The model under review builds one solid part; all positions refer to its coordinate system, in mm. Face numbers are marked on the shaded views. A direction names the side the tool comes from. Give positions to 0.01 mm unless a question says otherwise; leave off trailing zeros. Write each loop counter-clockwise with the first axis right and the second up, starting at its lowest first coordinate (ties: lowest second). Pieces come first, ordered by that corner, then holes. Notation, with made-up numbers: M 72,37 L 123,37 A7 ccw 123,46 Z; hole C 26.5,-21.75 d8. An arc over 180 degrees is marked long. Write item = value, one per line. Start each with the question number.
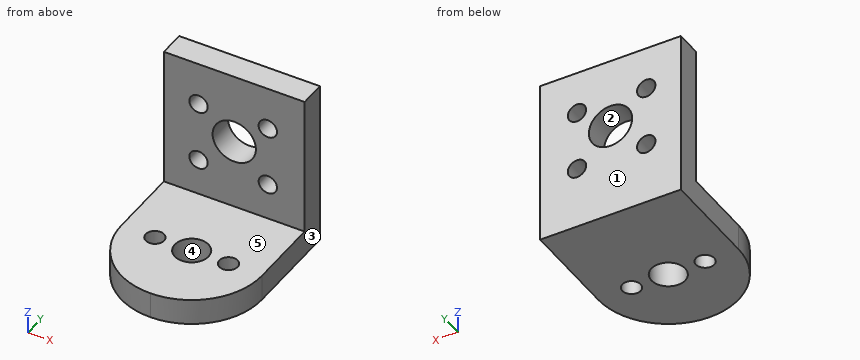
```python
from build123d import *

# Parameters (mm, degrees)
SKETCH1_W           = 32.5
SKETCH1_H           = 32.5
SKETCH1_R           = 2.125
SKETCH1_R_2         = 5
BOSS_EXTRUDE1_DEPTH = 6
SKETCH2_W           = 32.5
SKETCH2_H           = 6
BOSS_EXTRUDE2_DEPTH = 39
CUT_EXTRUDE1_DEPTH  = 39
SKETCH4_R           = 3.9
SKETCH4_R_2         = 2.125
CUT_EXTRUDE2_DEPTH  = 39


with BuildPart() as part:
    # Sketch1 → Boss-Extrude1 (new body)
    with BuildSketch(Plane(origin=(0, 0, 0), x_dir=(1, 0, 0), z_dir=(0, 1, 0))):
        with Locations((16.25, 16.25)):
            Rectangle(SKETCH1_W, SKETCH1_H)
        with Locations(Location((24, 10, 0), (0, 0, 270))):
            Circle(SKETCH1_R, mode=Mode.SUBTRACT)
        with Locations(Location((24, 24, 0), (0, 0, 270))):
            Circle(SKETCH1_R, mode=Mode.SUBTRACT)
        with Locations(Location((8, 24, 0), (0, 0, 270))):
            Circle(SKETCH1_R, mode=Mode.SUBTRACT)
        with Locations(Location((8, 10, 0), (0, 0, 270))):
            Circle(SKETCH1_R, mode=Mode.SUBTRACT)
        with Locations(Location((16.25, 16.25, 0), (0, 0, 270))):
            Circle(SKETCH1_R_2, mode=Mode.SUBTRACT)
    extrude(amount=BOSS_EXTRUDE1_DEPTH)

    # Sketch2 → Boss-Extrude2 (add)
    with BuildSketch(Plane(origin=(0, 6, 0), x_dir=(1, 0, 0), z_dir=(0, 1, 0))):
        with Locations((16.25, 35.5)):
            Rectangle(SKETCH2_W, SKETCH2_H)
    extrude(amount=-BOSS_EXTRUDE2_DEPTH)

    # Sketch3 → Cut-Extrude1 (cut)
    with BuildSketch(Plane.XY.offset(-32.5)):
        with BuildLine():
            Line((16.25, -33), (32.5, -33))
            Line((32.5, -33), (32.5, -16.75))
            ThreePointArc((32.5, -16.75), (27.740485194, -28.240485194), (16.25, -33))
        make_face()
        with BuildLine():
            Line((0, -33), (16.25, -33))
            ThreePointArc((16.25, -33), (4.759514806, -28.240485194), (0, -16.75))
            Line((0, -16.75), (0, -33))
        make_face()
    extrude(amount=-CUT_EXTRUDE1_DEPTH, mode=Mode.SUBTRACT)

    # Sketch4 → Cut-Extrude2 (cut)
    with BuildSketch(Plane.XY.offset(-32.5)):
        with Locations((16.25, -16.75)):
            Circle(SKETCH4_R)
        with Locations((7.75, -16.75)):
            Circle(SKETCH4_R_2)
        with Locations((24.75, -16.75)):
            Circle(SKETCH4_R_2)
    extrude(amount=-CUT_EXTRUDE2_DEPTH, mode=Mode.SUBTRACT)


solid = part.part
```
Item 1: For the marked faces 4 and 5, list the 3-axis set-ups (+Z, -Z, +X, -X, +Y, -Y) from which the entire face can be reached by the end or side of a thin tool; tool diameter is ignored.
Item 2: We need section B-B, the plane z = -16.25. Write out the cut boundary in (x, y), and give its area (3 significant figures).
Item 3: To check wall thickness, follow probe 1 along X at (y, z) = (4, -16.25); probe 2 along Y at (x, z) = (16, -35); probe 3 along X at (y, z) = (-17, -34). State the ranges of each line that lie inside material, in increasing order. Write a range as [from, to].
Item 4: Clearance check with flat-ended pins moving along their axes: P1, Ø10, axis at x = 9, y = -18, coming from the +Z side; P2, Ø16, axis at x = 8.5, z = -9, coming from the -Y side. State where each tip first meets the part, or that it passes through.
Item 5: We need section C-C, the plane x = 24. Write out the cut boundary in (y, z) (3 decimals), and give its area (3 significant figures).
Item 6: We need section D-D, the plane y = -13.5. Write out the cut boundary in (x, z), and give its area (3 significant figures).
Item 7: We need section A-A, the plane z = -24. Write out the cut boundary in (x, y) (3 decimals).
Item 8: The part is to be moulded in two halves that separate along X. For the marked faces 1, 2 and 3, say which applies: released by +X, released by -X, zero draft, split by the parting line, or undercut.
Worked out:
q1.face_4 = +Z, -Z
q1.face_5 = +Z, +X, -X, -Y
q2.outline = M 0,0 L 11.25,0 L 11.25,6 L 0,6 Z; M 21.25,0 L 32.5,0 L 32.5,6 L 21.25,6 Z
q2.area = 135 mm²
q3.probe_1 = [0, 11.25], [21.25, 32.5]
q3.probe_2 = [-33, -20.64], [-12.86, 6]
q3.probe_3 = [0, 5.64], [9.86, 12.36], [20.14, 22.64], [26.86, 32.5]
q4.P1 = -32.5
q4.P2 = 0
q5.outline = M -31.033,-38.5 L -18.738,-38.5 L -18.738,-32.5 L -31.033,-32.5 Z; M -14.762,-38.5 L 6,-38.5 L 6,-26.125 L 0,-26.125 L 0,-32.5 L -14.762,-32.5 Z; M 0,-21.875 L 6,-21.875 L 6,-12.125 L 0,-12.125 Z; M 0,-7.875 L 6,-7.875 L 6,0 L 0,0 Z
q5.area = 342 mm²
q6.outline = M 0,-38.5 L 14.09,-38.5 L 14.09,-32.5 L 0,-32.5 Z; M 18.41,-38.5 L 32.5,-38.5 L 32.5,-32.5 L 18.41,-32.5 Z
q6.area = 169 mm²
q7.outline = M 0,0 L 5.875,0 L 5.875,6 L 0,6 Z; M 10.125,0 L 21.875,0 L 21.875,6 L 10.125,6 Z; M 26.125,0 L 32.5,0 L 32.5,6 L 26.125,6 Z
q8.face_1 = zero draft
q8.face_2 = undercut
q8.face_3 = released by +X
